Verification items for the finished model (mm, model axes). A direction names the side the tool comes from. Coordinates: 2 decimals unless noted, no trailing zeros. Answer as a JSON object with one key per item and string values. Group by question number.
Q1. Release check for a two-part mould opening along Y. For faces 1 (the flat face through (0, -7.58, 39)), 2 (the flat face through (53, -5, -37.234)), 3 (the cylindrical face through (32, -8, -1)), 4 (the flat face through (0, 0, 36)) record: released by +Y, released by -Y, zero draft, split by the parting line, or undercut.
Q2. Gauge pin test, flat ends, axial feed: pin 1 Ø5 at (y, z) = (-7.5, -23) entering from +X; pin 2 Ø3 at (x, y) = (24, -2.5) entering from +Z; pin 3 Ø2 at (x, y) = (39, -1) entering from +Z. Record the tip position at first contact, or that the pin passes through.
Q3. Set-up check for faces 5 (the flat face through (50.5, -2.4, -34.234)), 6 (the flat face through (-30.283, -4.488, -0.217)), 7 (the cylindrical face through (32, -1, -1)), 8 (the flat face through (-2.655, -6.061, 38.562)): record each of +Z, -Z, +X, -X, +Y, -Y from which the full face is reachable in a straight line by a thin tool's end or side.
Q4. Scan lines: L1, parallel to Z at x = -6.5, y = -6; L2, parallel to X at y = -2.5, z = 21.5; L3, parallel to X at y = -3.25, z = -33. Record each from-to range of solid material in increasing order.
```python
from build123d import *

# Parameters (mm, degrees)
F1_DEPTH = 9
F2_R     = 3.429
F3_R     = 3.429
F4_DEPTH = 3
F6_DEPTH = 7.700001
F7_R     = 3.62132


with BuildPart() as f1:
    # F0 (on Front) → F1 (new body)
    with BuildSketch(Plane.XZ):
        Polygon((-10.932353, 34.76619), (0, 34.76619), (10.932353, 34.76619), (49.100234, -34.23381), (57.899766, -34.23381), (15.472571, 42.466191), (0, 42.466191), (-15.472571, 42.466191), (-57.899766, -34.23381), (-49.100234, -34.23381), align=None)
    extrude(amount=F1_DEPTH)

    # F2 (on face) + F3 (on face) → F4 (join)
    with BuildSketch(Plane(origin=(0, 0, -34.23381), x_dir=(1, 0, 0), z_dir=(0, 0, -1))):
        with Locations((-53.5, 4.5)):
            Circle(F2_R)
    with BuildSketch(Plane(origin=(0, 0, -34.23381), x_dir=(1, 0, 0), z_dir=(0, 0, -1))):
        with Locations((53.5, 4.5)):
            Circle(F3_R)
    extrude(amount=F4_DEPTH)

    # F5 (on face) → F6 (cut, through all)
    with BuildSketch(Plane(origin=(0, 0, 34.76619), x_dir=(1, 0, 0), z_dir=(0, 0, -1))):
        Polygon((-1.778, 7.579586), (-3.556, 4.5), (-1.778, 1.420414), (1.778, 1.420414), (3.556, 4.5), (1.778, 7.579586), align=None)
    extrude(amount=-F6_DEPTH, mode=Mode.SUBTRACT)

    # F7
    f7_edges = [f1.edges().sort_by_distance(p)[0] for p in [
        (-36.686169, -9, 4.11619),
        (-36.686169, 0, 4.11619),
        (36.686169, 0, 4.11619),
        (36.686169, -9, 4.11619),
        (-30.016294, -9, 0.26619),
        (-30.016294, 0, 0.26619),
        (30.016294, -9, 0.26619),
        (30.016294, 0, 0.26619),
    ]]
    fillet(f7_edges, radius=F7_R)


solid = f1.part
```
Computed values:
{
 "1": {"face 1": "undercut", "face 2": "zero draft", "face 3": "released by -Y", "face 4": "released by +Y"},
 "2": {"pin 1": "stops at x = 52.76", "pin 2": "stops at z = 29.52", "pin 3": "stops at z = 0.11"},
 "3": {"face 5": "-Z", "face 6": "-Z, +Y, -Y", "face 7": "-Z, +Y", "face 8": "+Z, -Z"},
 "4": {"L1": "z = 34.77 to 42.47", "L2": "x = -26.87 to -18.47, 18.47 to 26.87", "L3": "x = -57.2 to -48.44, 48.44 to 57.2"}
}
